Build history of the part. All positions in model axes, mm. A direction names the side the tool comes from. Round coordinates to 2 decimals unless told otherwise and drop trailing zeros. Loops run counter-clockwise (first coordinate to the right, second up) from the corner with the lowest first, then second, coordinate; pieces in that order, holes last. Notation, with made-up numbers: (77.5, -16.75) - (122.5, -16.75) arc R13 cw to (122.5, 3.25) - close; hole circle Ø7 at (58.5, 59.5). An arc over 180 degrees is marked (long way). Use one line per item in the form item = value. Start each with the question number.
Q1. Saw through at A-A (z = -35.5). Give the cut face in (x, y).
Q2. 3-axis set-ups, long thin cutter, end or side, ignore diameter. For faces 1 (the face through (105.88, 3.13, 47.35)), 2 (the face through (-124.833, 3.131, -1.416)), 3 (the face through (-16, 3.13, 27.13)): which of +Z, -Z, +X, -X, +Y, -Y reach the whole face in a straight line?
Q3. Saw through at D-D (x = 140). Give the cut face in (y, z), then the cut area to 3 significant figures.
Q4. Saw through at B-B (x = -141.5). Give the cut face in (y, z).
Q5. Saw through at C-C (y = 3). Count the separate pieces of the cut face and the enclosed holes in it, then the cut area to 3 significant figures.
Q6. Pin check, flat tips, straight feed: pin 1 (5 mm diameter, centred on x = 62.84, z = -56.52, fed in from +Y); pin 2 (1 mm diameter, centred on y = 1.5, z = -1, fed in from +X). Stop position of each tip, or through.
Q7. Mould opens along Z. For faces 4 (the face through (-116.5, 3.13, 62.83)), 5 (the face through (-185.882, 3.131, -60.043)), 6 (the face through (-3, 6.35, -17)) say: released by +Z, released by -Z, zero draft, split by the parting line, or undercut.
Q8. Drill centre lines: line 1 (X direction, y = 3.75, z = 10); line 2 (X direction, y = 4.75, z = 43); line 3 (X direction, y = 4.5, z = -59.5). Where is each one in solid material? Low to high.
```python
from build123d import *

# Parameters (mm, degrees)
SKETCH1_R           = 2.921
SKETCH1_R_2         = 2.2352
SKETCH1_R_3         = 12.3825
SKETCH1_R_4         = 10.8585
SKETCH1_R_5         = 14.0335
SKETCH1_R_6         = 1.7653
SKETCH1_R_7         = 40.0685
SKETCH1_R_8         = 1.9939
BOSS_EXTRUDE1_DEPTH = 6.35
SKETCH2_R           = 1.89865
CUT_EXTRUDE1_DEPTH  = 200.611442467
FILLET1_R           = 2.54


with BuildPart() as part:
    # Sketch1 → Boss-Extrude1 (new body)
    with BuildSketch(Plane(origin=(0, 0, 0), x_dir=(1, 0, 0), z_dir=(0, 1, 0))):
        with BuildLine():
            ThreePointArc((-173.185393891, 72.463962089), (-185.885393891, 59.763962089), (-173.185393891, 47.063962089))
            Line((-173.185393891, 47.063962089), (-149.978045472, 44.967655518))
            Line((-149.978045472, 44.967655518), (-98.053869436, -44.967655518))
            Line((-98.053869436, -44.967655518), (-110.525914692, -48.765439461))
            ThreePointArc((-110.525914692, -48.765439461), (-116.443172686, -63.050963961), (-104.175914692, -72.463962089))
            Line((-104.175914692, -72.463962089), (104.175914692, -72.463962089))
            ThreePointArc((104.175914692, -72.463962089), (116.443172686, -63.050963961), (110.525914692, -48.765439461))
            Line((110.525914692, -48.765439461), (98.053869436, -44.967655518))
            Line((98.053869436, -44.967655518), (149.978045472, 44.967655518))
            Line((149.978045472, 44.967655518), (173.185393891, 47.063962089))
            ThreePointArc((173.185393891, 47.063962089), (185.885393891, 59.763962089), (173.185393891, 72.463962089))
            Line((173.185393891, 72.463962089), (-173.185393891, 72.463962089))
        make_face()
        with Locations(Location((173.185393891, 59.763962089, 0), (0, 0, 270))):
            Circle(SKETCH1_R, mode=Mode.SUBTRACT)
        with Locations(Location((-104.175914692, -59.763962089, 0), (0, 0, 270))):
            Circle(SKETCH1_R, mode=Mode.SUBTRACT)
        with Locations(Location((-66.986243512, -59.763962089, 0), (0, 0, 270))):
            Circle(SKETCH1_R_2, mode=Mode.SUBTRACT)
        with Locations(Location((-66.986243512, -34.363962089, 0), (0, 0, 270))):
            Circle(SKETCH1_R_3, mode=Mode.SUBTRACT)
        with Locations(Location((-26.765079253, -28.544379147, 0), (0, 0, 270))):
            Circle(SKETCH1_R_4, mode=Mode.SUBTRACT)
        with Locations(Location((-66.986243512, -8.963962089, 0), (0, 0, 270))):
            Circle(SKETCH1_R_2, mode=Mode.SUBTRACT)
        with Locations(Location((16.020956488, -34.363962089, 0), (0, 0, 270))):
            Circle(SKETCH1_R_5, mode=Mode.SUBTRACT)
        with Locations(Location((81.81843836, -43.438397329, 0), (0, 0, 270))):
            Circle(SKETCH1_R_6, mode=Mode.SUBTRACT)
        with Locations(Location((-173.185393891, 59.763962089, 0), (0, 0, 270))):
            Circle(SKETCH1_R, mode=Mode.SUBTRACT)
        with Locations(Location((72.790674122, 4.112206637, 0), (0, 0, 270))):
            Circle(SKETCH1_R_7, mode=Mode.SUBTRACT)
        with Locations(Location((35.857528241, 46.975232392, 0), (0, 0, 270))):
            Circle(SKETCH1_R_2, mode=Mode.SUBTRACT)
        with Locations(Location((62.841482041, 56.516110851, 0), (0, 0, 270))):
            Circle(SKETCH1_R_8, mode=Mode.SUBTRACT)
        with Locations(Location((91.444570369, 57.528762089, 0), (0, 0, 270))):
            Circle(SKETCH1_R_2, mode=Mode.SUBTRACT)
        with Locations(Location((133.608398757, 56.516110851, 0), (0, 0, 270))):
            Circle(SKETCH1_R_8, mode=Mode.SUBTRACT)
        with Locations(Location((104.175914692, -59.763962089, 0), (0, 0, 270))):
            Circle(SKETCH1_R, mode=Mode.SUBTRACT)
    extrude(amount=BOSS_EXTRUDE1_DEPTH)

    # Sketch2 → Cut-Extrude1 (cut, through all)
    with BuildSketch(Plane(origin=(0, 6.35, 0), x_dir=(1, 0, 0), z_dir=(0, 1, 0))):
        with Locations(Location((-99.282752504, 46.975232392, 0), (0, 0, 270))):
            Circle(SKETCH2_R)
        with Locations(Location((-26.765079253, 46.975232392, 0), (0, 0, 270))):
            Circle(SKETCH2_R)
        with Locations(Location((-3.029043512, -59.670924273, 0), (0, 0, 270))):
            Circle(SKETCH2_R)
        with Locations(Location((-1.772813917, 13.610193745, 0), (0, 0, 270))):
            Circle(SKETCH2_R)
    extrude(amount=-CUT_EXTRUDE1_DEPTH, mode=Mode.SUBTRACT)

    # Fillet1
    fillet1_edges = [part.edges().sort_by_distance(p)[0] for p in [
        (149.978045472, 3.175, -44.967655518),
        (98.053869436, 3.175, 44.967655518),
        (-98.053869436, 3.175, 44.967655518),
        (-149.978045472, 3.175, -44.967655518),
    ]]
    fillet(fillet1_edges, radius=FILLET1_R)


solid = part.part
```
Report:
q1.outline = (-144.51, 0) - (47.89, 0) - (47.89, 6.35) - (-144.51, 6.35) - close; (97.7, 0) - (144.51, 0) - (144.51, 6.35) - (97.7, 6.35) - close
q2.face_1 = +X, +Y, -Y
q2.face_2 = -X, +Y, -Y
q2.face_3 = +Y, -Y
q3.outline = (0, -72.46) - (6.35, -72.46) - (6.35, -27.69) - (0, -27.69) - close
q3.area = 284 mm²
q4.outline = (0, -72.46) - (6.35, -72.46) - (6.35, -30.28) - (0, -30.28) - close
q5.separate_pieces = 1
q5.enclosed_holes = 19
q5.area = 31,800 mm²
q6.pin_1 = 6.35
q6.pin_2 = 124.88
q7.face_4 = undercut
q7.face_5 = split by the parting line
q7.face_6 = zero draft
q8.line_1 = -118.24 to -68.97, -65.01 to 35.29, 110.29 to 118.24
q8.line_2 = -99.36 to -75.86, -58.11 to 4.96, 27.08 to 80.11, 83.53 to 99.36
q8.line_3 = -185.88 to -176.09, -170.28 to 90.39, 92.5 to 170.28, 176.09 to 185.88
